```python
from build123d import *

# Parameters (mm, degrees)
CHAMFER1_SIZE                = 0.5
SKETCH2_R                    = 2
CUT_EXTRUDE1_DEPTH           = 6.5
CIRPATTERN1_COUNT            = 3
SKETCH3_R                    = 2
BOSS_EXTRUDE1_DEPTH          = 3
CHAMFER2_SIZE                = 0.1
CIRPATTERN3_COUNT            = 3
CHAMFER2_OF_CIRPATTERN3_SIZE = 0.1


with BuildPart() as part:
    # Sketch1 → Revolve1 (revolve)
    with BuildSketch(Plane.XY, mode=Mode.PRIVATE) as revolve1_sk:
        Polygon((-22.25, 0), (-22.25, 5), (-16.25, 5), (-16.25, 7), (16.25, 7), (16.25, 21), (22.75, 21), (22.75, 0), align=None)
    revolve(revolve1_sk.sketch.rotate(Axis((-54.078202457, 0, 0), (1, 0, 0)), 90), axis=Axis((-54.078202457, 0, 0), (1, 0, 0)))

    # Chamfer1
    chamfer1_edges = [part.edges().sort_by_distance(p)[0] for p in [
        (22.75, 0, -21),
    ]]
    chamfer(chamfer1_edges, length=CHAMFER1_SIZE)

    # Sketch2 → Cut-Extrude1 (cut)
    with BuildSketch(Plane(origin=(22.75, 0, 0), x_dir=(0, 0, -1), z_dir=(1, 0, 0))):
        with Locations((0, 15)):
            Circle(SKETCH2_R)
    cut_extrude1 = extrude(amount=-CUT_EXTRUDE1_DEPTH, mode=Mode.SUBTRACT)

    # CirPattern1: Cut-Extrude1 ×3 about axis
    cirpattern1_axis = Axis((0, 0, 0), (1, 0, 0))
    for i in range(1, CIRPATTERN1_COUNT):
        add(cut_extrude1.rotate(cirpattern1_axis, i * 360 / CIRPATTERN1_COUNT), mode=Mode.SUBTRACT)

    # Sketch3 → Boss-Extrude1 (add)
    with BuildSketch(Plane(origin=(22.75, 0, 0), x_dir=(0, 0, -1), z_dir=(1, 0, 0))):
        with Locations(Location((12.340862004, 7.125, 0), (0, 0, 180))):
            Circle(SKETCH3_R)
    boss_extrude1 = extrude(amount=BOSS_EXTRUDE1_DEPTH)

    # Chamfer2
    chamfer2_edges = [part.edges().sort_by_distance(p)[0] for p in [
        (25.75, 7.125, -14.340862004),
    ]]
    chamfer(chamfer2_edges, length=CHAMFER2_SIZE)

    # CirPattern3: Boss-Extrude1 ×3 about axis
    cirpattern3_axis = Axis((0, 0, 0), (1, 0, 0))
    for i in range(1, CIRPATTERN3_COUNT):
        add(boss_extrude1.rotate(cirpattern3_axis, i * 360 / CIRPATTERN3_COUNT))

    # Chamfer2 of CirPattern3
    chamfer2_of_cirpattern3_edges = [part.edges().sort_by_distance(p)[0] for p in [
        (25.75, 8.857050808, 13.340862004),
        (25.75, -15.982050808, 1),
    ]]
    chamfer(chamfer2_of_cirpattern3_edges, length=CHAMFER2_OF_CIRPATTERN3_SIZE)


solid = part.part
```
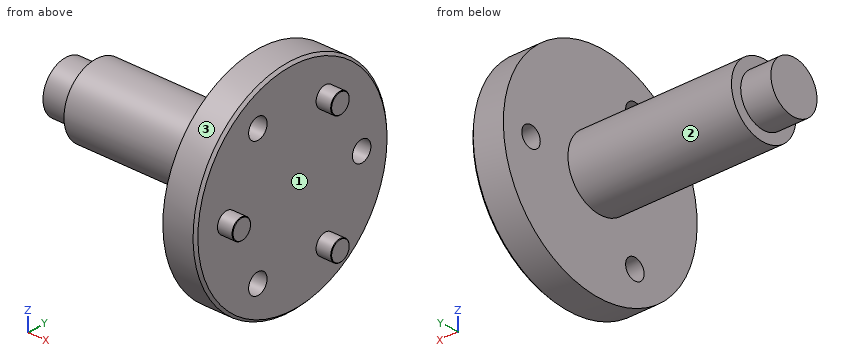
Source: CAD feature listing. Evaluate the final solid. Frame: model axes, mm. Face numbers are marked on the shaded views. A direction names the side the tool comes from. Round coordinates to 2 decimals unless told otherwise and drop trailing zeros. Loops run counter-clockwise (first coordinate to the right, second up) from the corner with the lowest first, then second, coordinate; pieces in that order, holes last. Notation, with made-up numbers: M 68,15 L 97,15 A13 cw 97,36 Z; hole C -16,-28.75 d11. An arc over 180 degrees is marked long. Use a Markdown table: item, result. Add a question column.
1. Section query D-D on x = -2. Return the cut outline in (y, z).
2. Section query A-A on z = 0. Return the cut outline in (x, y), then the cut area to 3 significant figures.
3. Reachability of the marked faces 1, 2 and 3 from +Z, -Z, +X, -X, +Y, -Y: full face, straight path, thin tool, end or side. Return the list, or none.
4. Section query B-B on y = 0. Return the cut outline in (x, z).
5. Section query C-C on x = 20.5. Return the cut outline in (y, z).
6. Line query: line 1 (X direction, y = -4.5, z = 11); line 2 (Y direction, x = 18, z = 0); line 3 (Y direction, x = 20.5, z = 13). Output: solid intervals per line, ascending.
7. Contact query for flat-ended pins moving along their axis: P1, Ø5, axis at y = 15, z = 0, coming from the +X side; P2, Ø5, axis at x = 18.5, y = 6, coming from the +Z side; P3, Ø10, axis at x = 10, y = -4, coming from the +Z side; P4, Ø3.5, axis at y = -7.5, z = -12.99, coming from the +X side. Output: stop coordinate, or through.
Reported:
| question | item | result |
|---|---|---|
| 1 | outline | C 0,0 d14 |
| 2 | outline | M -22.25,-5 L -16.25,-5 L -16.25,-7 L 16.25,-7 L 16.25,-21 L 22.25,-21 L 22.75,-20.5 L 22.75,-16.25 L 25.65,-16.25 L 25.75,-16.15 L 25.75,-12.35 L 25.65,-12.25 L 22.75,-12.25 L 22.75,13 L 16.25,13 L 16.25,7 L -16.25,7 L -16.25,5 L -22.25,5 Z; M 16.25,17 L 22.75,17 L 22.75,20.5 L 22.25,21 L 16.25,21 Z |
| 2 | area | 774 mm² |
| 3 | face 1 | +X |
| 3 | face 2 | -X |
| 3 | face 3 | +X, -X |
| 4 | outline | M -22.25,-5 L -16.25,-5 L -16.25,-7 L 16.25,-7 L 16.25,-21 L 22.25,-21 L 22.75,-20.5 L 22.75,20.5 L 22.25,21 L 16.25,21 L 16.25,7 L -16.25,7 L -16.25,5 L -22.25,5 Z |
| 5 | outline | C 0,0 d42; hole C -7.5,-12.99 d4; hole C -7.5,12.99 d4; hole C 15,0 d4 |
| 6 | line 1 | x = 16.25 to 22.75 |
| 6 | line 2 | y = -21 to 13, 17 to 21 |
| 6 | line 3 | y = -16.49 to -9.5, -5.5 to 16.49 |
| 7 | P1 | stops at x = 22.75 |
| 7 | P2 | stops at z = 20.71 |
| 7 | P3 | stops at z = 7 |
| 7 | P4 | passes through |
